Can you work these out from the model? Positions are in its coordinate system, mm. Face numbers are marked on the shaded views. A direction names the side the tool comes from. Coordinates: 2 decimals unless noted, no trailing zeros. Order: outer loops, then holes, each group sorted by start corner. A loop starts at its lowest first (then second) coordinate and runs counter-clockwise, first axis right, second up. Notation, with made-up numbers: (78, -17.75) - (104, -17.75) arc R24 cw to (104, -5.75) - close; hole circle Ø10 at (9.5, -22.5). An arc over 180 degrees is marked (long way). Use a Markdown table: item, result. Add a question column.
(1) On a 3-axis mill with a long thin cutter (end or side, diameter ignored), from which of +Z, -Z, +X, -X, +Y, -Y can I reach the whole of each face in a straight line? I mean the marked faces 4, 5 and 6. Say none if no direction works.
(2) I want a section at B-B (z = 2.75). List the corners of the cut face in (x, y) for me, and give its area (3 significant figures).
(3) For pin 1 Ø1.5 at (x, y) = (-15.5, 1) entering from +Z; pin 2 Ø3 at (x, z) = (-16.5, 3) entering from +Y; pin 3 Ø1 at (y, z) = (-2.5, -1.5) entering from +X; pin 4 Ø1.5 at (y, z) = (-2, 1.5) entering from +X, each with a flat end and sliding along its axis, tell me the tip position at first contact or that it passes through.
(4) I want a section at C-C (x = -14.75). List the corners of the cut face in (y, z) for me, and give its area (3 significant figures).
(5) I want a section at D-D (y = -2.5). List the corners of the cut face in (x, z) for me.
(6) I want a section at A-A (y = 0). List the corners of the cut face in (x, z) for me, and give its area (3 significant figures).
(7) We'd pull the mould along Y, two halves only. Please class the marked faces 1, 2 and 3: pulls with the +Y half, pulls with the -Y half, needs draft (parallel to the pull), parting line crosses it, or undercut.
(8) If I drill on L1, parallel to X at y = -1.25, z = 0.5; L2, parallel to X at y = 0.5, z = 3.25; L3, parallel to Z at x = 0.25, y = 3, over which ranges is the centre line in solid material (lowest first)? Write a range as [from, to].
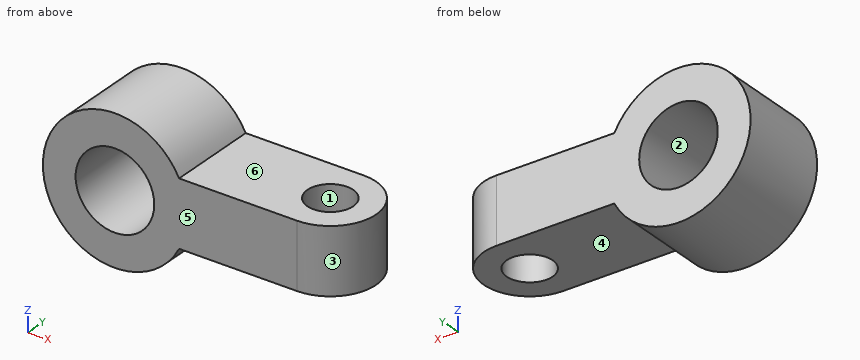
```python
from build123d import *

# Parameters (mm, degrees)
ESBO_O1_R                = 1.75
RESSALTO_EXTRUS_O1_DEPTH = 5
ESBO_O2_R                = 3
RESSALTO_EXTRUS_O2_DEPTH = 7


with BuildPart() as part:
    # Esboço1 → Ressalto-extrusão1 (new body)
    with BuildSketch(Plane.XY):
        with BuildLine():
            Line((0, 3.5), (-6, 3.5))
            Line((-6, 3.5), (-6, -3.5))
            Line((-6, -3.5), (0, -3.5))
            ThreePointArc((0, -3.5), (3.5, 0), (0, 3.5))
        make_face()
        Circle(ESBO_O1_R, mode=Mode.SUBTRACT)
    extrude(amount=RESSALTO_EXTRUS_O1_DEPTH)

    # Esboço2 → Ressalto-extrusão2 (add)
    with BuildSketch(Plane(origin=(0, 3.5, 0), x_dir=(1, 0, 0), z_dir=(0, 1, 0))):
        with BuildLine():
            Line((-6, -5), (-6, 0))
            Line((-6, 0), (-9, 0))
            ThreePointArc((-9, 0), (-19.398979486, -2.5), (-9, -5))
            Line((-9, -5), (-6, -5))
        make_face()
        with Locations((-13.898979486, -2.5)):
            Circle(ESBO_O2_R, mode=Mode.SUBTRACT)
    extrude(amount=-RESSALTO_EXTRUS_O2_DEPTH)


solid = part.part
```
Answers follow:
| question | item | result |
|---|---|---|
| 1 | face 4 | -Z, +X, +Y, -Y |
| 1 | face 5 | +Z, -Z, +X, -X, -Y |
| 1 | face 6 | +Z, +X, +Y, -Y |
| 2 | outline | (-19.39, -3.5) - (-16.89, -3.5) - (-16.89, 3.5) - (-19.39, 3.5) - close; (-10.91, -3.5) - (0, -3.5) arc R3.5 ccw to (0, 3.5) - (-10.91, 3.5) - close; hole circle Ø3.5 at (0, 0) |
| 2 | area | 104 mm² |
| 3 | pin 1 | stops at z = 7.93 |
| 3 | pin 2 | stops at y = 3.5 |
| 3 | pin 3 | stops at x = -9.66 |
| 3 | pin 4 | stops at x = 3.27 |
| 4 | outline | (-3.5, -2.93) - (3.5, -2.93) - (3.5, -0.38) - (-3.5, -0.38) - close; (-3.5, 5.38) - (3.5, 5.38) - (3.5, 7.93) - (-3.5, 7.93) - close |
| 4 | area | 35.8 mm² |
| 5 | outline | (-9, 0) - (2.45, 0) - (2.45, 5) - (-9, 5) arc R5.5 ccw (long way) to start; hole circle Ø6 at (-13.9, 2.5) |
| 6 | outline | (-9, 0) - (-1.75, 0) - (-1.75, 5) - (-9, 5) arc R5.5 ccw (long way) to start; (1.75, 0) - (3.5, 0) - (3.5, 5) - (1.75, 5) - close; hole circle Ø6 at (-13.9, 2.5) |
| 6 | area | 110 mm² |
| 7 | face 1 | undercut |
| 7 | face 2 | needs draft |
| 7 | face 3 | parting line crosses it |
| 8 | L1 | x = [-19.02, -16.14], [-11.66, -1.22], [1.22, 3.27] |
| 8 | L2 | x = [-19.35, -16.8], [-10.99, -1.68], [1.68, 3.46] |
| 8 | L3 | z = [0, 5] |
